Check sheet for the drawn part. Datum: minimum x, y, z corner. Units: mm. Coordinates: 2 decimals unless noted, no trailing zeros. Write each loop counter-clockwise with the first axis right and the second up, starting at its lowest first coordinate (ties: lowest second). Pieces come first, ordered by that corner, then holes. Notation, with made-up numbers: (57, 17.5) - (70, 17.5) arc R21 ccw to (70, 28.5) - close; hole circle Ø2 at (-38, 1.25). An arc over 180 degrees is marked (long way). Write each question's results on one line, items separated by ' | '.
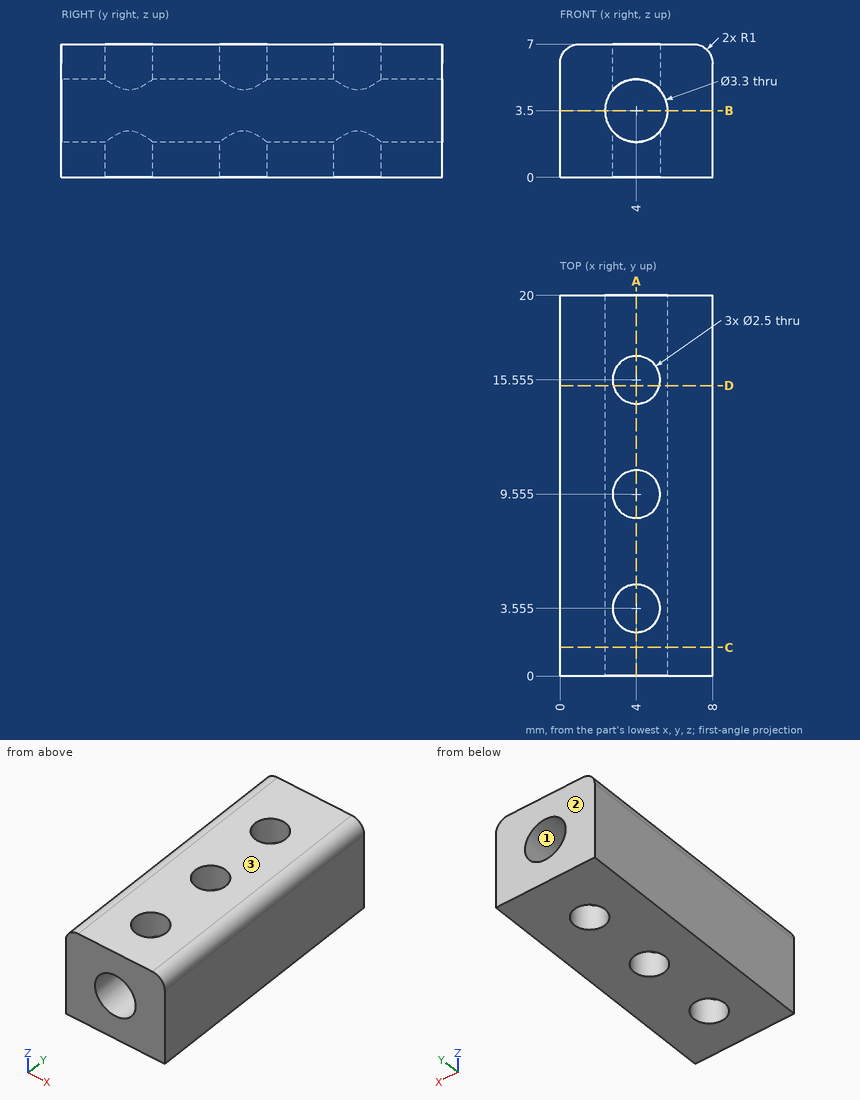
1. Sectioned sample at D-D (y = 15.25). Record the cut outline in (x, z).
Values follow:
outline: (0, 0) - (2.79, 0) - (2.79, 2.38) arc R1.65 cw to (2.79, 4.62) - (2.79, 7) - (1, 7) arc R1 ccw to (0, 6) - close; (5.21, 0) - (8, 0) - (8, 6) arc R1 ccw to (7, 7) - (5.21, 7) - (5.21, 4.62) arc R1.65 cw to (5.21, 2.38) - close
2. Sectioned sample at B-B (z = 3.5). Record the cut outline in (x, y).
Values follow:
outline: (0, 0) - (2.35, 0) - (2.35, 20) - (0, 20) - close; (5.65, 0) - (8, 0) - (8, 20) - (5.65, 20) - close
3. Draft check along Z on the marked faces 1, 2 and 3. Enter one of: pulls with the +Z half, pulls with the -Z half, needs draft (parallel to the pull), parting line crosses it, or undercut.
Values follow:
face 1: undercut | face 2: needs draft | face 3: pulls with the +Z half
4. Sectioned sample at A-A (x = 4). Give the number of separate pieces and of enclosed holes in the cut face, then the cut area to 4 significant figures.
Values follow:
separate pieces: 8 | enclosed holes: 0 | area: 46.25 mm^2
5. Sectioned sample at C-C (y = 1.5). Record the cut outline in (x, z).
Values follow:
outline: (0, 0) - (8, 0) - (8, 6) arc R1 ccw to (7, 7) - (1, 7) arc R1 ccw to (0, 6) - close; hole circle Ø3.3 at (4, 3.5)
6. Material ranges on L1, parallel to Y at x = 4, z = 5.55 (3 decimals); L2, parallel to Y at x = 3, z = 6 (3 decimals); L3, parallel to Z at x = 4, y = 5.5, recorded low to high. Write a range as [from, to].
Values follow:
L1: y = [0, 2.305], [4.805, 8.305], [10.805, 14.305], [16.805, 20] | L2: y = [0, 2.805], [4.305, 8.805], [10.305, 14.805], [16.305, 20] | L3: z = [0, 1.85], [5.15, 7]
